Geometry check sheet. Reference: the model listing, model coordinates, mm. A direction names the side the tool comes from. Coordinates: 2 decimals unless noted, no trailing zeros. Write each loop counter-clockwise with the first axis right and the second up, starting at its lowest first coordinate (ties: lowest second). Pieces come first, ordered by that corner, then holes. Notation, with made-up numbers: (12.25, 45.25) -> (53.25, 45.25) arc R24 cw to (53.25, 66.25) -> close; hole circle Ø2 at (-36, -34). An arc over 180 degrees is marked (long way). One line per question, with ' | ' between items.
```python
from build123d import *

# Parameters (mm, degrees)
F0_W     = 10
F0_H     = 16
F1_DEPTH = 2
F3_DEPTH = 2


# Not quite as in the source:
# - ends of sketch curves that miss each other by under 0.0002 mm in the source are joined


with BuildPart() as f1:
    # F0 (on Top) → F1 (new body)
    with BuildSketch(Plane.XY):
        Rectangle(F0_W, F0_H)
    extrude(amount=F1_DEPTH)

    # F2 (on face) → F3 (join)
    with BuildSketch(Plane.XY.offset(2)):
        Polygon((0, 7), (-2, 7), (-3, 6), (-2, 5), (0, 5), (2, 5), (3, 6), (2, 7), align=None)
        Polygon((2, 0.891659756), (2.00782e-05, 0.9006214721), (-2, 0.891659756), (-3, 0), (-2, -0.891659756), (-2.00782e-05, -0.9006214721), (2, -0.891659756), (3, 0), align=None)
        Polygon((0, -5), (-2, -5), (-3, -6), (-2, -7), (0, -7), (2, -7), (3, -6), (2, -5), align=None)
        Polygon((-4.1414213562, -4.8585786438), (-3.1414213562, -5.8585786438), (-2.1414213562, -4.8585786438), (-2.1414213562, -1.0335195075), (-3.1374518146, -0.1453992321), (-4.1414213562, -1.1507223826), align=None)
        Polygon((4.1414213562, 4.8585786438), (3.1414213562, 5.8585786438), (2.1414213562, 4.8585786438), (2.1414213562, 1.0335195075), (3.1374518146, 0.1453992321), (4.1414213562, 1.1507223826), align=None)
    extrude(amount=F3_DEPTH)


solid = f1.part
```
(1) Draft check along Y on faces 1 (the face through (3, 3, 4)), 2 (the face through (-2.141, -3, 3)), 3 (the face through (0, -7, 3)), 4 (the face through (0, 2, 2)). Enter one of: pulls with the +Y half, pulls with the -Y half, needs draft (parallel to the pull), parting line crosses it, or undercut.
Answers below:
face 1: needs draft | face 2: undercut | face 3: pulls with the -Y half | face 4: undercut
(2) Cross-section at B-B (y = -3.25). Record the cut outline in (x, z).
Answers below:
outline: (-5, 0) -> (5, 0) -> (5, 2) -> (-2.14, 2) -> (-2.14, 4) -> (-4.14, 4) -> (-4.14, 2) -> (-5, 2) -> close
(3) Tool access check on faces 5 (the face through (2.5, 5.5, 3)), 6 (the face through (2.5, 6.5, 3)), 7 (the face through (2.493, -0.452, 2.986)). Record the directions out of +Z, -Z, +X, -X, +Y, -Y that give a thin tool (end or side, any length) a straight path to the whole face; none if there is none.
Answers below:
face 5: +Z | face 6: +Z, +X, +Y | face 7: +Z, +X
(4) Cross-section at D-D (y = 6.5). Record the cut outline in (x, z), plus the area to 3 significant figures.
Answers below:
outline: (-5, 0) -> (5, 0) -> (5, 2) -> (2.5, 2) -> (2.5, 4) -> (-2.5, 4) -> (-2.5, 2) -> (-5, 2) -> close | area: 30.0 mm²
(5) Cross-section at A-A (z = 2.85). Count the separate pieces of the cut face and the enclosed holes in it, plus the area to 3 significant figures.
Answers below:
separate pieces: 5 | enclosed holes: 0 | area: 47.9 mm²
(6) Cross-section at C-C (x = -0.5). Record the cut outline in (y, z).
Answers below:
outline: (-8, 0) -> (8, 0) -> (8, 2) -> (7, 2) -> (7, 4) -> (5, 4) -> (5, 2) -> (0.9, 2) -> (0.9, 4) -> (-0.9, 4) -> (-0.9, 2) -> (-5, 2) -> (-5, 4) -> (-7, 4) -> (-7, 2) -> (-8, 2) -> close
(7) Depth check by flat-ended pin: P1, Ø0.6, axis at y = 3.5, z = 3.5, coming from the -X side; P2, Ø1.5, axis at y = 3, z = 3, coming from the +X side; P3, Ø1.6, axis at y = -3, z = 3.5, coming from the -X side. Enter the tip coordinate at first touch or a pass-through.
Answers below:
P1: stops at x = 2.14 | P2: stops at x = 4.14 | P3: stops at x = -4.14
(8) Material ranges on line 1 (Y direction, x = 1.75, z = 3.65); line 2 (X direction, y = 3.25, z = 3); line 3 (Z direction, x = 3, y = -3.5), recorded low to high.
Answers below:
line 1: y = -7 to -5, -0.89 to 0.89, 5 to 7 | line 2: x = 2.14 to 4.14 | line 3: z = 0 to 2
